Geometry check sheet. Reference: the model listing, model coordinates, mm. Give positions to 0.01 mm unless a question says otherwise; leave off trailing zeros. Order: outer loops, then holes, each group sorted by start corner. A loop starts at its lowest first (then second) coordinate and runs counter-clockwise, first axis right, second up.
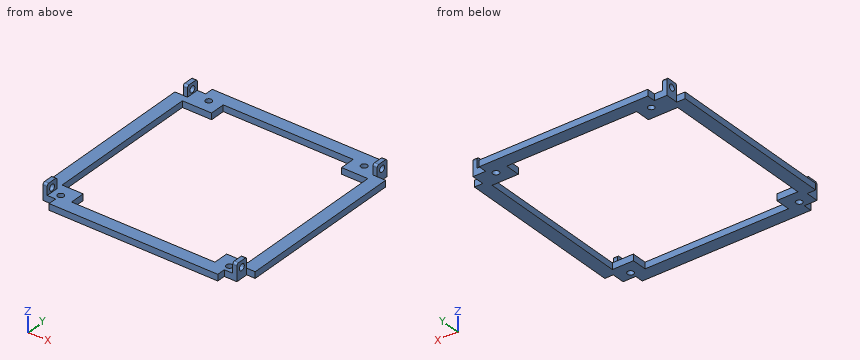
Solid Edge part; units mm, degrees
sketch "Sketch1" plane through (0, 0, 0) normal (0, 0, 1) x (1, 0, 0)
  line L0 (-40, -50) -> (40, -50)
  line L1 (40, -50) -> (50, -50)
  line L2 (50, -50) -> (50, -40)
  line L3 (50, -40) -> (50, 40)
  line L4 (50, 50) -> (50, 40)
  line L5 (40, 50) -> (50, 50)
  line L6 (40, 50) -> (-40, 50)
  line L7 (-50, 50) -> (-40, 50)
  line L8 (-50, 40) -> (-50, 50)
  line L9 (-50, 40) -> (-50, -40)
  line L10 (-50, -40) -> (-50, -50)
  line L11 (-50, -50) -> (-40, -50)
extrude "Protrusion1" add sketch "Sketch1" against normal blind 5
sketch "Sketch2" plane through (0, 0, 0) normal (0, 0, 1) x (1, 0, 0)
  line L0 (50, 50) -> (40, 50)
  line L1 (40, 46) -> (40, 50)
  line L2 (40, 46) -> (46, 46)
  line L3 (46, 46) -> (46, 40)
  line L4 (46, 40) -> (50, 40)
  line L5 (50, 40) -> (50, 50)
  line L6 (50, -40) -> (50, -50)
  line L7 (50, -50) -> (40, -50)
  line L8 (40, -46) -> (40, -50)
  line L9 (46, -46) -> (40, -46)
  line L10 (46, -40) -> (46, -46)
  line L11 (46, -40) -> (50, -40)
  line L12 (-50, -50) -> (-40, -50)
  line L13 (-40, -46) -> (-40, -50)
  line L14 (-46, -46) -> (-40, -46)
  line L15 (-46, -40) -> (-46, -46)
  line L16 (-50, -40) -> (-46, -40)
  line L17 (-50, -40) -> (-50, -50)
  line L18 (-46, 40) -> (-46, 46)
  line L19 (-46, 46) -> (-40, 46)
  line L20 (-40, 46) -> (-40, 50)
  line L21 (-40, 50) -> (-50, 50)
  line L22 (-50, 50) -> (-50, 40)
  line L23 (-50, 40) -> (-46, 40)
  dimension "D1" = 40
  dimension "D2" = 40
  dimension "D3" = 50
  dimension "D4" = 50
  dimension "D5" = 50
  dimension "D6" = 50
  dimension "D7" = 40
  dimension "D8" = 46
  dimension "D9" = 46
  dimension "D10" = 50
  dimension "D11" = 50
  dimension "D12" = 40
  dimension "D13" = 50
  dimension "D14" = 50
  dimension "D15" = 50
  dimension "D16" = 40
extrude "ExtrudedCutout_1" cut sketch "Sketch2" against normal blind 11.3526
sketch "Sketch3" plane through (0, 0, 0) normal (0, 0, 1) x (1, 0, 0)
  circle A0 centre (-40, -42.86) radius 1.5
  circle A1 centre (-36.13, 42.87) radius 1.5
  circle A2 centre (40, -42.86) radius 1.5
  circle A3 centre (37.53, 42.87) radius 1.5
extrude "Cutout1" cut sketch "Sketch3" against normal blind 5
sketch "Sketch4" plane through (0, 0, 0) normal (0, 0, 1) x (0, 1, 0)
  line L0 (36.87, 44) -> (-36.86, 44)
  line L1 (-36.86, 44) -> (-36.86, 34)
  line L2 (-36.86, 34) -> (-44, 34)
  line L3 (-44, 34) -> (-44, -34)
  line L4 (-44, -34) -> (-36.86, -34)
  line L5 (-36.86, -34) -> (-36.86, -44)
  line L6 (-36.86, -44) -> (36.87, -44)
  line L7 (36.87, -44) -> (36.87, -31.53)
  line L8 (36.87, -31.53) -> (44, -31.53)
  line L9 (44, -31.53) -> (44, 30.13)
  line L10 (44, 30.13) -> (36.87, 30.13)
  line L11 (36.87, 30.13) -> (36.87, 44)
extrude "Cutout2" cut sketch "Sketch4" against normal blind 5
sketch "Sketch5" plane through (0, 0, 0) normal (0, 0, 1) x (1, 0, 0)
  line L0 (-46, 40) -> (-44, 40)
  line L1 (-44, 40) -> (-44, 46)
  line L2 (-44, 46) -> (-46, 46)
  line L3 (-46, 40) -> (-46, 46)
  line L4 (46, 46) -> (44, 46)
  line L5 (44, 46) -> (44, 40)
  line L6 (44, 40) -> (46, 40)
  line L7 (46, 40) -> (46, 46)
  line L8 (-46, -40) -> (-44, -40)
  line L9 (-44, -40) -> (-44, -46)
  line L10 (-44, -46) -> (-46, -46)
  line L11 (-46, -46) -> (-46, -40)
  line L12 (46, -46) -> (44, -46)
  line L13 (44, -46) -> (44, -40)
  line L14 (44, -40) -> (46, -40)
  line L15 (46, -40) -> (46, -46)
extrude "ExtrudedProtrusion_3" add sketch "Sketch5" along normal blind 5
sketch "Sketch6" plane through (-44, -43, 3) normal (1, 0, 0) x (0, 1, 0)
  circle A0 centre (0, -1) radius 1.5
  circle A1 centre (85.9991, -1) radius 1.5
extrude "ExtrudedCutout_14" cut sketch "Sketch6" against normal blind 2
sketch "Sketch7" plane through (44, 43, 2.5) normal (-1, 0, 0) x (0, -1, 0)
  circle A0 centre (0.0009, -0.5) radius 1.5
  circle A1 centre (86, -0.5) radius 1.5
extrude "ExtrudedCutout_15" cut sketch "Sketch7" against normal blind 2
fillet "Round_2" radius 1 8 edges at (45, 40, 5) (45, 46, 5) (-45, 40, 5) (-45, 46, 5) (-45, -46, 5) (-45, -40, 5) (45, -46, 5) (45, -40, 5)
sketch "Sketch8" plane through (0, 0, -5) normal (0, 0, -1) x (0, -1, 0)
  line L0 (-50, -50) -> (50, -50)
  line L1 (50, -50) -> (50, 50)
  line L2 (50, 50) -> (-50, 50)
  line L3 (-50, 50) -> (-50, -50)
  dimension "D1" = 50
  dimension "D2" = 50
extrude "ExtrudedCutout_16" cut sketch "Sketch8" against normal blind 2
Item 1: Sectioned sample at D-D (y = -42.86). Enter the section's corners in (x, z).
Reported:
outline: (-46, -3) - (-41.5, -3) - (-41.5, 0) - (-44, 0) - (-44, 0.51) - (-46, 0.51) - close; (-46, 3.49) - (-44, 3.49) - (-44, 5) - (-46, 5) - close; (-38.5, -3) - (-34, -3) - (-34, 0) - (-38.5, 0) - close; (34, -3) - (38.5, -3) - (38.5, 0) - (34, 0) - close; (41.5, -3) - (46, -3) - (46, 0.51) - (44, 0.51) - (44, 0) - (41.5, 0) - close; (44, 3.49) - (46, 3.49) - (46, 5) - (44, 5) - close
Item 2: Sectioned sample at A-A (z = 2). Give the number of separate pieces and of enclosed holes in the cut face, and give its area (3 significant figures).
Reported:
separate pieces: 8
enclosed holes: 0
area: 24.0 mm2
Item 3: Scan lines: L1, parallel to Y at x = -36.13, z = -0.8; L2, parallel to X at y = -43, z = -0.25; L3, parallel to Y at x = -12.5, z = -2.25. Record each from-to range of solid material in increasing order.
Reported:
L1: y = -50 to -36.86, 36.87 to 41.37, 44.37 to 50
L2: x = -46 to -41.49, -38.51 to -34, 34 to 38.51, 41.49 to 46
L3: y = -50 to -44, 44 to 50
Item 4: Sectioned sample at B-B (x = 11.5). Enter the section's corners in (y, z), and give its area (3 significant figures).
Reported:
outline: (-50, -3) - (-44, -3) - (-44, 0) - (-50, 0) - close; (44, -3) - (50, -3) - (50, 0) - (44, 0) - close
area: 36.0 mm2
Item 5: Gauge pin test, flat ends, axial feed: pin 1 (2.5 mm diameter, centred on x = -36.13, y = 42.87, fed in from +Z); pin 2 (3.5 mm diameter, centred on y = 48, z = -1, fed in from -X); pin 3 (1.8 mm diameter, centred on x = -43.5, z = 1, fed in from -Y); pin 4 (1.5 mm diameter, centred on x = 48, z = -1, fed in from -Y). Record the tip position at first contact, or that the pin passes through.
Reported:
pin 1: passes through
pin 2: stops at x = -40
pin 3: stops at y = -46
pin 4: stops at y = -40
